The model under review builds one solid part; all positions refer to its coordinate system, in mm. A direction names the side the tool comes from. Round coordinates to 2 decimals unless told otherwise and drop trailing zeros. Write each loop counter-clockwise with the first axis right and the second up, starting at its lowest first coordinate (ties: lowest second). Pieces come first, ordered by that corner, then holes. Notation, with made-up numbers: (-39.75, 55) -> (-7.75, 55) arc R13 cw to (-7.75, 78) -> close; hole circle Ø6 at (-9.75, 61.25). An arc over 180 degrees is marked (long way). Use CSV: the item, a comma, the result in double quotes. Start each with the question number.
1) Machinability: for faces 1 (the face through (44.959, 3, 92)), 2 (the face through (70.359, 3, 92)), 3 (the face through (45.518, 3, 80)), 4 (the face through (44.959, 3, 3)), 5 (the face through (83.059, 3, 3)), which of the approach directions +Z, -Z, +X, -X, +Y, -Y give a long, thin tool a straight path to every point of the face, cutting with its end or side? Answer none if there is none.
2) Wall thickness on probe 1 along Z at (x, y) = (75.5, 0.5); probe 2 along X at (y, z) = (2.5, 82.55); probe 3 along Z at (x, y) = (114.5, 0.5): over which ranges is each line inside the solid? List them lowest first. Write a range as [from, to].
3) Mouldability with a two-part tool opening along Z and no side actions: class faces 6 (the face through (38.306, 3, 63)), 7 (the face through (45.518, 3, 13)), 8 (the face through (104, 3, 0)) as released by +Z, released by -Z, zero draft, split by the parting line, or undercut.
4) Take a section at D-D, the plane y = 3.5. State how many separate pieces and enclosed holes the cut face has, then the cut area to 3 significant figures.
5) Take a section at B-B, the plane x = 98. Give the boundary of the cut face in (y, z).
6) Take a section at C-C, the plane z = 12.7. Give the boundary of the cut face in (x, y), then the cut area to 3 significant figures.
7) Take a section at A-A, the plane z = 23.5. Give the boundary of the cut face in (x, y).
8) For pin 1 Ø1.5 at (x, y) = (59, 1.5) entering from -Z; pin 2 Ø1.9 at (x, y) = (64.5, 2.5) entering from +Z; pin 3 Ø3 at (x, z) = (133.54, 9.68) entering from +Y; pin 4 Ø3 at (y, z) = (3, 14.5) entering from -X, all flat-tipped, find the tip position at first contact; note any pin that passes through.
from build123d import *

# Parameters (mm, degrees)
SKETCH2_W           = 120.952956328
SKETCH2_H           = 6.35
BOSS_EXTRUDE1_DEPTH = 95.25
SKETCH3_R           = 39.37
CUT_EXTRUDE2_DEPTH  = 7.35
CUT_EXTRUDE3_DEPTH  = 7.35
SKETCH5_W           = 31.75
SKETCH5_H           = 25.4
CUT_EXTRUDE4_DEPTH  = 7.35
SKETCH6_W           = 12.7
SKETCH6_H           = 6.35
CUT_EXTRUDE5_DEPTH  = 7.35
LPATTERN1_COUNT     = 3
LPATTERN1_PITCH     = 25.4
SKETCH7_W           = 7.21259173
SKETCH7_H           = 12.7
SKETCH7_H_2         = 19.05
CUT_EXTRUDE6_DEPTH  = 7.35
SKETCH8_R           = 1.75
CUT_EXTRUDE7_DEPTH  = 7.35
SKETCH10_R          = 1.75
CUT_EXTRUDE9_DEPTH  = 7.35


with BuildPart() as part:
    # Sketch2 → Boss-Extrude1 (new body)
    with BuildSketch(Plane.XY):
        with Locations((98.782063621, 3.175)):
            Rectangle(SKETCH2_W, SKETCH2_H)
    extrude(amount=BOSS_EXTRUDE1_DEPTH)

    # Sketch3 → Cut-Extrude2 (cut, through all)
    with BuildSketch(Plane(origin=(0, 6.35, 0), x_dir=(1, 0, 0), z_dir=(0, 1, 0))):
        with Locations((111.633541785, -47.625)):
            Circle(SKETCH3_R)
    extrude(amount=-CUT_EXTRUDE2_DEPTH, mode=Mode.SUBTRACT)

    # Sketch4 → Cut-Extrude3 (cut, through all)
    with BuildSketch(Plane(origin=(0, 6.35, 0), x_dir=(1, 0, 0), z_dir=(0, 1, 0))):
        with BuildLine():
            Line((111.633541785, -95.25), (179.051442703, -95.25))
            Line((179.051442703, -95.25), (179.051442703, 0))
            Line((179.051442703, 0), (111.633541785, 0))
            ThreePointArc((111.633541785, 0), (159.258541785, -47.625), (111.633541785, -95.25))
        make_face()
    extrude(amount=-CUT_EXTRUDE3_DEPTH, mode=Mode.SUBTRACT)

    # Sketch5 → Cut-Extrude4 (cut, through all)
    with BuildSketch(Plane(origin=(0, 6.35, 0), x_dir=(1, 0, 0), z_dir=(0, 1, 0))):
        with Locations((54.180585457, -31.75)):
            Rectangle(SKETCH5_W, SKETCH5_H)
    extrude(amount=-CUT_EXTRUDE4_DEPTH, mode=Mode.SUBTRACT)

    # Sketch6 → Cut-Extrude5 (cut, through all)
    with BuildSketch(Plane(origin=(0, 6.35, 0), x_dir=(1, 0, 0), z_dir=(0, 1, 0))):
        with Locations((89.408541785, -3.175)):
            Rectangle(SKETCH6_W, SKETCH6_H)
        with Locations((89.408541785, -92.075)):
            Rectangle(SKETCH6_W, SKETCH6_H)
    cut_extrude5 = extrude(amount=-CUT_EXTRUDE5_DEPTH, mode=Mode.SUBTRACT)

    # LPattern1: Cut-Extrude5 ×3
    with Locations(*[(-i * LPATTERN1_PITCH, 0, 0) for i in range(1, LPATTERN1_COUNT)]):
        add(cut_extrude5, mode=Mode.SUBTRACT)

    # Sketch7 → Cut-Extrude6 (cut, through all)
    with BuildSketch(Plane(origin=(0, 6.35, 0), x_dir=(1, 0, 0), z_dir=(0, 1, 0))):
        with Locations((41.911881322, -12.7)):
            Rectangle(SKETCH7_W, SKETCH7_H)
        with Locations((41.911881322, -79.375)):
            Rectangle(SKETCH7_W, SKETCH7_H_2)
        with Locations((41.911881322, -50.8)):
            Rectangle(SKETCH7_W, SKETCH7_H)
    extrude(amount=-CUT_EXTRUDE6_DEPTH, mode=Mode.SUBTRACT)

    # Sketch8 → Cut-Extrude7 (cut, through all)
    with BuildSketch(Plane(origin=(0, 6.35, 0), x_dir=(1, 0, 0), z_dir=(0, 1, 0))):
        with Locations((76.708541785, -12.7)):
            Circle(SKETCH8_R)
        with Locations((76.708541785, -82.55)):
            Circle(SKETCH8_R)
    extrude(amount=-CUT_EXTRUDE7_DEPTH, mode=Mode.SUBTRACT)

    # Sketch10 → Cut-Extrude9 (cut, through all)
    with BuildSketch(Plane(origin=(0, 6.35, 0), x_dir=(1, 0, 0), z_dir=(0, 1, 0))):
        with Locations((133.541041785, -9.680096933)):
            Circle(SKETCH10_R)
    extrude(amount=-CUT_EXTRUDE9_DEPTH, mode=Mode.SUBTRACT)


solid = part.part
Values found:
1,face 1,"+Z, -X, +Y, -Y"
1,face 2,"+Z, +Y, -Y"
1,face 3,"-X, +Y, -Y"
1,face 4,"-Z, -X, +Y, -Y"
1,face 5,"-Z, +Y, -Y"
2,probe 1,"[0, 11.43], [13.97, 31.99], [63.26, 81.28], [83.82, 95.25]"
2,probe 2,"[45.52, 74.96], [78.46, 93.46], [129.81, 144.01]"
2,probe 3,"[0.09, 8.36], [86.89, 95.16]"
3,face 6,"zero draft"
3,face 7,"undercut"
3,face 8,"released by -Z"
4,separate pieces,"1"
4,enclosed holes,"4"
4,area,"4,110 mm²"
5,outline,"(0, 0) -> (6.35, 0) -> (6.35, 10.69) -> (0, 10.69) -> close; (0, 84.56) -> (6.35, 84.56) -> (6.35, 95.25) -> (0, 95.25) -> close"
6,outline,"(45.52, 0) -> (74.96, 0) -> (74.96, 6.35) -> (45.52, 6.35) -> close; (78.46, 0) -> (93.46, 0) -> (93.46, 6.35) -> (78.46, 6.35) -> close; (129.81, 0) -> (144.01, 0) -> (144.01, 6.35) -> (129.81, 6.35) -> close"
6,area,"372 mm²"
7,outline,"(70.06, 0) -> (80.52, 0) -> (80.52, 6.35) -> (70.06, 6.35) -> close; (142.75, 0) -> (152.7, 0) -> (152.7, 6.35) -> (142.75, 6.35) -> close"
8,pin 1,"z = 6.35"
8,pin 2,"z = 88.9"
8,pin 3,"through"
8,pin 4,"x = 45.52"
